Check sheet for the modelled part. Datum: model origin and axes. Units: mm. A direction names the side the tool comes from. Round coordinates to 2 decimals unless told otherwise and drop trailing zeros. Order: outer loops, then holes, each group sorted by start corner. A loop starts at its lowest first (then second) coordinate and runs counter-clockwise, first axis right, second up.
Autodesk Inventor part; units mm, degrees
ref_plane "YZ Plane" through (0, 0, 0) normal (1, 0, 0) x (0, 1, 0)
ref_plane "XZ Plane" through (0, 0, 0) normal (0, 1, 0) x (-1, 0, 0)
ref_plane "XY Plane" through (0, 0, 0) normal (0, 0, 1) x (1, 0, 0)
sketch "Szkic10" plane through (0, 0, 0) normal (0, 1, 0) x (-1, 0, 0)
  line L0 (-25, 60) -> (25, 60)
  line L1 (25, 60) -> (25, -60)
  line L2 (25, -60) -> (-25, -60)
  line L3 (-25, -60) -> (-25, 60)
  line L4 (-25, 60) -> (25, -60) construction
  line L5 (25, 60) -> (-25, -60) construction
  point P0 (0, 0)
  dimension "d75" = 50
  dimension "d76" = 120
extrude "Wyciągnięcie proste6" add sketch "Szkic10" along normal blind 10
sketch "Szkic11" plane through (-25, 0, -60) normal (-1, 0, 0) x (0, 0, 1)
  line L0 (120, 0) -> (0, 0)
  line L1 (120, 0) -> (120, 10)
  line L2 (0, 10) -> (120, 10)
  line L3 (0, 0) -> (0, 10)
  line L4 (0, 0) -> (120, 0)
  line L5 (0, 0) -> (0, 5)
  line L6 (0, 5) -> (120, 5)
  line L7 (0, 5) -> (20, 5)
  line L8 (20, 5) -> (40, 5)
  line L9 (40, 5) -> (80, 5)
  line L10 (80, 5) -> (100, 5)
  circle A0 centre (20, 5) radius 2.5
  circle A1 centre (40, 5) radius 2.5
  circle A2 centre (80, 5) radius 2.5
  circle A3 centre (100, 5) radius 2.5
  point P0 (60, 0)
  dimension "d79" = 5
  dimension "d80" = 20
  dimension "d81" = 20
  dimension "d84" = 5
  dimension "d85" = 5
  dimension "d86" = 5
  dimension "d87" = 5
  dimension "d105" = 20
  dimension "d106" = 20
extrude "Wyciągnięcie proste7" cut sketch "Szkic11" against normal blind 20 contours A3 L6 | L6 A3 | A0 L6 | L6 A0 | A2 L6 | L6 A2 | A1 L6 | L6 A1
sketch "Szkic12" plane through (0, 10, 0) normal (0, 1, 0) x (1, 0, 0)
  line L0 (25, -60) -> (25, 60)
  line L1 (25, 0) -> (3, 0)
  circle A0 centre (3, 0) radius 15
  point P0 (0, 0)
  dimension "d102" = 22
  dimension "d103" = 30
extrude "Wyciągnięcie proste8" cut sketch "Szkic12" against normal up to next
sketch "Szkic13" plane through (0, 0, 0) normal (0, -1, 0) x (1, 0, 0)
  line L0 (25, 60) -> (-25, 60)
  line L1 (-25, 60) -> (-25, -60)
  line L2 (-25, -60) -> (25, -60)
  line L3 (25, -60) -> (25, 60)
  line L4 (25, 60) -> (25, 50)
  line L5 (25, -60) -> (25, 60)
  line L6 (25, 50) -> (-25, 50)
  line L7 (25, -60) -> (25, -50)
  line L8 (25, -50) -> (-25, -50)
  line L9 (25, 50) -> (15, 50)
  line L10 (25, -50) -> (15, -50)
  circle A0 centre (15, 50) radius 5
  circle A1 centre (15, -50) radius 5
  point P0 (0, 0)
  dimension "d93" = 10
  dimension "d94" = 10
  dimension "d95" = 10
  dimension "d96" = 10
  dimension "d97" = 10
  dimension "d98" = 10
extrude "Wyciągnięcie proste9" cut sketch "Szkic13" against normal blind 3 contours A0 L6 | L6 A0 | A1 L8 | L8 A1
sketch "Szkic14" plane through (15, 3, -50) normal (0, -1, 0) x (1, 0, 0)
  circle A0 centre (0, 0) radius 5
  circle A1 centre (0, 100) radius 5
  point P0 (-15, 50)
extrude "Wyciągnięcie proste10" cut sketch "Szkic14" against normal blind 10
sketch "Szkic15" plane through (25, 0, 60) normal (1, 0, 0) x (0, 0, -1)
  line L0 (120, 0) -> (0, 0)
  line L1 (120, 0) -> (120, 10)
  line L2 (0, 10) -> (120, 10)
  line L3 (0, 0) -> (0, 10)
  point P0 (60, 0)
extrude "Wyciągnięcie proste11" add sketch "Szkic15" along normal blind 7
sketch "Szkic16" plane through (-25, 0, 60) normal (0, 0, 1) x (1, 0, 0)
  line L0 (57, 0) -> (0, 0)
  line L1 (57, 10) -> (57, 0)
  line L2 (0, 10) -> (57, 10)
  line L3 (0, 0) -> (0, 10)
  line L4 (35, 10) -> (45, 10)
  line L5 (45, 0) -> (35, 0)
  line L6 (53, 0) -> (45, 0)
  line L7 (57, 0) -> (0, 0)
  line L8 (45, 0) -> (45, 10)
  line L9 (0, 10) -> (57, 10)
  line L10 (57, 10) -> (57, 0)
  line L11 (53, 5) -> (45, 5)
  line L12 (45, 5) -> (49, 5)
  circle A0 centre (49, 5) radius 2
  line L13 (49, 5) -> (53, 5)
  line L14 (53, 5) -> (53, 10)
  line L15 (53, 5) -> (53, 0)
  point P0 (25, 0)
  dimension "d113" = 4
  dimension "d114" = 4
  dimension "d115" = 5
  dimension "d116" = 45
  dimension "d117" = 4
sketch "Szkic17" plane through (-25, 0, -60) normal (0, 0, -1) x (-1, 0, 0)
  line L0 (-53, 10) -> (0, 10)
  line L1 (-53, 0) -> (-53, 10)
  line L2 (0, 0) -> (-53, 0)
  line L3 (0, 10) -> (0, 0)
  line L4 (-35, 0) -> (-45, 0)
  line L5 (-45, 10) -> (-35, 10)
  line L6 (-53, 10) -> (-45, 10)
  line L7 (-53, 10) -> (0, 10)
  line L8 (-45, 10) -> (-45, 0)
  line L9 (0, 0) -> (-53, 0)
  line L10 (-53, 0) -> (-53, 10)
  line L11 (-53, 5) -> (-45, 5)
  line L12 (-45, 5) -> (-49, 5)
  circle A0 centre (-49, 5) radius 2
  line L13 (-49, 5) -> (-53, 5)
  line L14 (-53, 5) -> (-53, 0)
  line L15 (-53, 5) -> (-53, 10)
  line L16 (0, 0) -> (-57, 0)
  line L17 (0, 0) -> (0, 10)
  point P0 (-25, 0)
  point P1 (-25, 10)
  dimension "d119" = 4
  dimension "d120" = 4
  dimension "d121" = 5
  dimension "d122" = 45
  dimension "d123" = 4
hole "Otwór4" at (24, 5, -60) direction (0, 0, 1) diameter 4 depth 20 tip angle 118
hole "Otwór5" at (24, 5, 60) direction (0, 0, -1) diameter 4 depth 20 tip angle 118
sketch "Szkic18" plane through (0, 0, 0) normal (0, -1, 0) x (1, 0, 0)
  circle A0 centre (15, -50) radius 5
  circle A1 centre (15, 50) radius 5
  circle A2 centre (3, 0) radius 15
  line L0 (32, 60) -> (-25, 60)
  line L1 (-25, 60) -> (-25, -60)
  line L2 (-25, -60) -> (32, -60)
  line L3 (32, 60) -> (32, -60)
  line L4 (15, -50) -> (32, -50)
  line L5 (15, 50) -> (32, 50)
  line L6 (32, -60) -> (32, 60)
  line L7 (15, 50) -> (15, 51.5)
  line L8 (15, 51.5) -> (32, 51.5)
  line L9 (15, 50) -> (15, 48.5)
  line L10 (15, 48.5) -> (32, 48.5)
  line L11 (15, -50) -> (15, -48.5)
  line L12 (15, -48.5) -> (32, -48.5)
  line L13 (15, -50) -> (15, -51.5)
  line L14 (15, -51.5) -> (32, -51.5)
  point P0 (0, 0)
  dimension "d138" = 1.5
  dimension "d139" = 1.5
  dimension "d140" = 1.5
  dimension "d141" = 1.5
extrude "Wyciągnięcie proste12" cut sketch "Szkic18" against normal up to next contours L4 L11 L12 A0 | L4 L3 L14 A0 | A0 L14 L13 L4 | A0 L12 L3 L4 | L10 A1 L5 L3 | L5 A1 L8 L3 | L10 L9 L5 A1 | L5 L7 L8 A1
thread "Gwint9"
thread "Gwint10"
thread "Gwint11"
thread "Gwint12"
properties part number "Podstawa dolna osi Z"
1) Sectioned sample at B-B on z = 0. Record the cut outline in (x, y).
2) Gauge pin test, flat ends, axial feed: pin 1 (3.5 mm diameter, centred on x = 24, y = 5, fed in from +Z); pin 2 (3.5 mm diameter, centred on x = 24, y = 5, fed in from -Z); pin 3 (3 mm diameter, centred on y = 5, z = -40, fed in from -X). Record the tip position at first contact, or that the pin passes through.
3) Sectioned sample at A-A on x = 15. Record the cut outline in (y, z), and give its area (3 significant figures).
4) Scan lines: line 1 (Z direction, x = -12.75, y = 5); line 2 (X direction, y = 5, z = -55.75); line 3 (Y direction, x = -16.5, z = -20). Record each from-to range of solid material in increasing order.
5) Sectioned sample at C-C on x = 3. Record the cut outline in (y, z).
6) Set-up check for faces 1 (the face through (24, 3, -56)), 2 (the face through (22.648, 6.474, 44.19)), 3 (the face through (-15.14, 4.04, 42.31)), 4 (the face through (26, 4, -48.5)): record each of +Z, -Z, +X, -X, +Y, -Y from which the full face is reachable in a straight line by a thin tool's end or side.
7) Sectioned sample at D-D on x = -19. Record the cut outline in (y, z), and give its area (3 significant figures).
8) Draft check along Z on faces 5 (the face through (3, 5, 60)), 6 (the face through (22.648, 6.474, 55.69)), 7 (the face through (-5, 5, 20)). Enter one of: pulls with the +Z half, pulls with the -Z half, needs draft (parallel to the pull), parting line crosses it, or undercut.
Values found:
1. outline: (-25, 0) - (-12, 0) - (-12, 10) - (-25, 10) - close; (18, 0) - (32, 0) - (32, 10) - (18, 10) - close
2. pin 1: stops at z = 39.85
2. pin 2: stops at z = -39.85
2. pin 3: stops at x = -5
3. outline: (0, -60) - (10, -60) - (10, -55) - (0, -55) - close; (0, -45) - (10, -45) - (10, -9) - (0, -9) - close; (0, 9) - (10, 9) - (10, 45) - (0, 45) - close; (0, 55) - (10, 55) - (10, 60) - (0, 60) - close
3. area: 820 mm2
4. line 1: z = -60 to -42.5, -37.5 to -22.5, -17.5 to 17.5, 22.5 to 37.5, 42.5 to 60
4. line 2: x = -25 to 22, 26 to 32
4. line 3: y = 0 to 2.5, 7.5 to 10
5. outline: (0, -60) - (10, -60) - (10, -15) - (0, -15) - close; (0, 15) - (10, 15) - (10, 60) - (0, 60) - close
6. face 1: -Z
6. face 2: +Z
6. face 3: -X
6. face 4: +X, +Y, -Y
7. outline: (0, -60) - (10, -60) - (10, 60) - (0, 60) - close; hole circle Ø5 at (5, -40); hole circle Ø5 at (5, -20); hole circle Ø5 at (5, 20); hole circle Ø5 at (5, 40)
7. area: 1,120 mm2
8. face 5: pulls with the +Z half
8. face 6: needs draft
8. face 7: undercut
